from build123d import *

# Parameters (mm, degrees)
SKETCH1_R           = 1.5
BOSS_EXTRUDE1_DEPTH = 10


with BuildPart() as part:
    # Sketch1 → Boss-Extrude1 (new body)
    with BuildSketch(Plane.XY):
        with BuildLine():
            Line((-1.84, -26.94), (-1.84, -4.476605857))
            ThreePointArc((-1.84, -4.476605857), (0, -4.84), (1.84, -4.476605857))
            Line((1.84, -4.476605857), (1.84, -26.94))
            ThreePointArc((1.84, -26.94), (2.718679656, -29.061320344), (4.84, -29.94))
            Line((4.84, -29.94), (19.84, -29.94))
            Line((19.84, -29.94), (19.84, -26.94))
            Line((19.84, -26.94), (7.84, -26.94))
            ThreePointArc((7.84, -26.94), (5.718679656, -26.061320344), (4.84, -23.94))
            Line((4.84, -23.94), (4.84, 0))
            ThreePointArc((4.84, 0), (0, 4.84), (-4.84, 0))
            Line((-4.84, 0), (-4.84, -23.94))
            ThreePointArc((-4.84, -23.94), (-5.718679656, -26.061320344), (-7.84, -26.94))
            Line((-7.84, -26.94), (-19.84, -26.94))
            Line((-19.84, -26.94), (-19.84, -29.94))
            Line((-19.84, -29.94), (-4.84, -29.94))
            ThreePointArc((-4.84, -29.94), (-2.718679656, -29.061320344), (-1.84, -26.94))
        make_face()
        Circle(SKETCH1_R, mode=Mode.SUBTRACT)
    extrude(amount=BOSS_EXTRUDE1_DEPTH)


solid = part.part
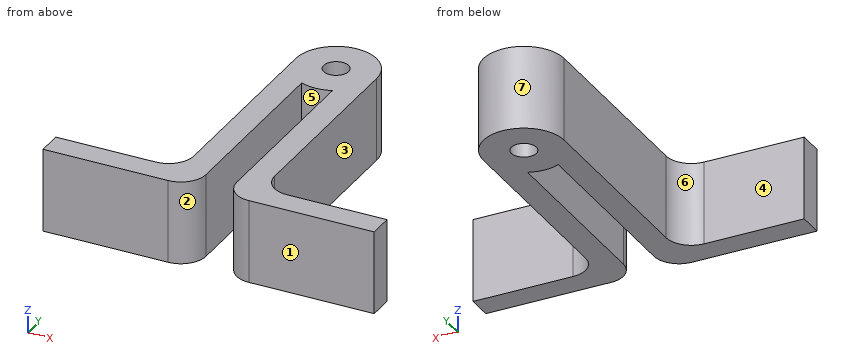
Source: CAD feature listing. Evaluate the final solid. Frame: model axes, mm. Face numbers are marked on the shaded views. A direction names the side the tool comes from. Coordinates: 2 decimals unless noted, no trailing zeros. Order: outer loops, then holes, each group sorted by start corner. A loop starts at its lowest first (then second) coordinate and runs counter-clockwise, first axis right, second up.
Item 1: Cut plane B-B (x = 0). Return loops of the section in (y, z).
Output values:
outline: (-4.84, 0) - (-1.5, 0) - (-1.5, 10) - (-4.84, 10) - close; (1.5, 0) - (4.84, 0) - (4.84, 10) - (1.5, 10) - close
Item 2: First-contact query: P1, Ø4, axis at y = -0.5, z = 5.5, coming from the -X side; P2, Ø1, axis at x = 4, z = 5.5, coming from the +Y side; P3, Ø3, axis at y = -9, z = 6.5, coming from the +X side. Flat tips, straight axial feed; report the tip coordinate or a pass-through.
Output values:
P1: stops at x = -4.84
P2: stops at y = 3.34
P3: stops at x = 4.84
Item 3: Material intervals for line 1 (X direction, y = -18.5, z = 9.25); line 2 (Y direction, x = 0, z = 2.5); line 3 (X direction, y = -2, z = 0.5), sorted ascending.
Output values:
line 1: x = -4.84 to -1.84, 1.84 to 4.84
line 2: y = -4.84 to -1.5, 1.5 to 4.84
line 3: x = -4.84 to 4.84
Item 4: Cut plane A-A (y = -22). Return loops of the section in (x, z).
Output values:
outline: (-4.84, 0) - (-1.84, 0) - (-1.84, 10) - (-4.84, 10) - close; (1.84, 0) - (4.84, 0) - (4.84, 10) - (1.84, 10) - close
Item 5: Pull-direction query (X, two-part tool) for the marked faces 5, 6 and 7; classes: pulls with the +X half, pulls with the -X half, needs draft (parallel to the pull), parting line crosses it, or undercut.
Output values:
face 5: undercut
face 6: pulls with the -X half
face 7: parting line crosses it
Item 6: Set-up query: the marked faces 1, 2, 3 and 4. Return all of +Z, -Z, +X, -X, +Y, -Y with unobstructed straight access to the full face (end or side cutting, diameter ignored); none if empty.
Output values:
face 1: +Z, -Z, +X, -X, -Y
face 2: +Z, -Z, -Y
face 3: +Z, -Z, +X, +Y
face 4: +Z, -Z, -X, +Y
Item 7: Cut plane C-C (z = 1). Return loops of the section in (x, y).
Output values:
outline: (-19.84, -29.94) - (-4.84, -29.94) arc R3 ccw to (-1.84, -26.94) - (-1.84, -4.48) arc R4.84 ccw to (1.84, -4.48) - (1.84, -26.94) arc R3 ccw to (4.84, -29.94) - (19.84, -29.94) - (19.84, -26.94) - (7.84, -26.94) arc R3 cw to (4.84, -23.94) - (4.84, 0) arc R4.84 ccw to (-4.84, 0) - (-4.84, -23.94) arc R3 cw to (-7.84, -26.94) - (-19.84, -26.94) - close; hole circle Ø3 at (0, 0)
Item 8: Cut plane D-D (x = -15). Return loops of the section in (y, z), plus the area to 3 significant figures.
Output values:
outline: (-29.94, 0) - (-26.94, 0) - (-26.94, 10) - (-29.94, 10) - close
area: 30.0 mm2
